```python
from build123d import *

# Parameters (mm, degrees)
SKETCH1_R           = 12
BOSS_EXTRUDE1_DEPTH = 31
FILLET1_R           = 1
SKETCH2_R           = 11.5
CUT_EXTRUDE1_DEPTH  = 1
SKETCH3_R           = 12.25
BOSS_EXTRUDE2_DEPTH = 20
FILLET2_R           = 0.5
SKETCH4_R           = 3.5
BOSS_EXTRUDE3_DEPTH = 3
SKETCH5_R           = 1.125510402
BOSS_EXTRUDE4_DEPTH = 9.5


with BuildPart() as part:
    # Sketch1 → Boss-Extrude1 (new body)
    with BuildSketch(Plane(origin=(0, 0, 0), x_dir=(0, 0, -1), z_dir=(1, 0, 0))):
        Circle(SKETCH1_R)
    extrude(amount=BOSS_EXTRUDE1_DEPTH)

    # Fillet1
    fillet1_edges = [part.edges().sort_by_distance(p)[0] for p in [
        (31, 0, 12),
    ]]
    fillet(fillet1_edges, radius=FILLET1_R)

    # Sketch2 → Cut-Extrude1 (cut)
    with BuildSketch(Plane.ZY):
        Circle(SKETCH2_R)
    extrude(amount=-CUT_EXTRUDE1_DEPTH, mode=Mode.SUBTRACT)

    # Sketch3 → Boss-Extrude2 (add)
    with BuildSketch(Plane(origin=(31, 0, 0), x_dir=(0, 0, -1), z_dir=(1, 0, 0))):
        Circle(SKETCH3_R)
    extrude(amount=BOSS_EXTRUDE2_DEPTH)

    # Fillet2
    fillet2_edges = [part.edges().sort_by_distance(p)[0] for p in [
        (31, 0, 12.25),
        (51, 0, 12.25),
    ]]
    fillet(fillet2_edges, radius=FILLET2_R)

    # Sketch4 → Boss-Extrude3 (add)
    with BuildSketch(Plane(origin=(51, 0, 0), x_dir=(0, 0, -1), z_dir=(1, 0, 0))):
        Circle(SKETCH4_R)
    extrude(amount=BOSS_EXTRUDE3_DEPTH)

    # Sketch5 → Boss-Extrude4 (add)
    with BuildSketch(Plane(origin=(54, 0, 0), x_dir=(0, 0, -1), z_dir=(1, 0, 0))):
        Circle(SKETCH5_R)
    extrude(amount=BOSS_EXTRUDE4_DEPTH)


solid = part.part
```
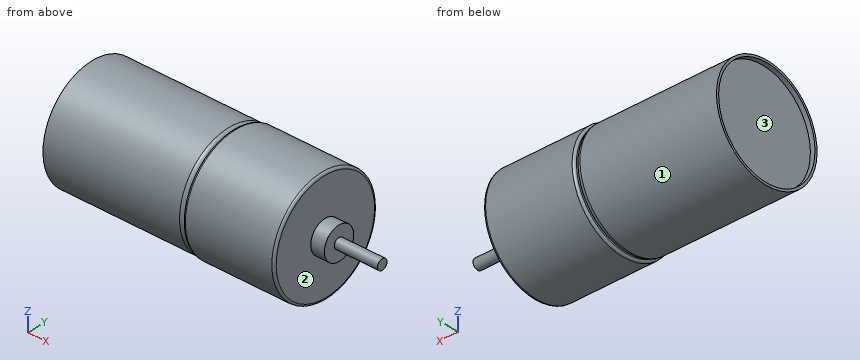
For this review, take the finished solid that the model builds, in its own axes (mm). Face numbers are marked on the shaded views. Give positions to 0.01 mm unless a question says otherwise; leave off trailing zeros. Loops run counter-clockwise (first coordinate to the right, second up) from the corner with the lowest first, then second, coordinate; pieces in that order, holes last. Notation, with made-up numbers: M -12.5,22 L 22.5,22 A34 ccw 22.5,58 Z; hole C 51,23.25 d1. An arc over 180 degrees is marked long. One line per item, written item: value. Start each with the question number.
Q1. Clearance check with flat-ended pins moving along their axes: pin 1 Ø10 at (y, z) = (9, 6) entering from +X; pin 2 Ø5 at (x, z) = (32.5, 3) entering from +Y; pin 3 Ø4 at (x, z) = (17, 0) entering from +Y. State where each tip first meets the part, or that it passes through.
Q2. For L1, parallel to Y at x = 0.3, z = 0; L2, parallel to X at y = 8, z = -5; L3, parallel to X at y = 0.5, z = 0.5, list the stretches that pass through material, from the lowest coordinate up.
Q3. Draft analysis for pull direction Y (two halves, no side actions). For the marked faces 1, 2 and 3, state which applies: released by +Y, released by -Y, zero draft, split by the parting line, or undercut.
Q4. Add section A-A (y = 0). Give the boundary of the cut face in (x, z), and give its area (3 significant figures).
Q5. Add section C-C (x = 8.5). Give the boundary of the cut face in (y, z).
Q6. Add section D-D (x = 56.5). Give the boundary of the cut face in (y, z), and give its area (3 significant figures).
Reply:
1. pin 1: x = 51
1. pin 2: y = 12.24
1. pin 3: y = 12
2. L1: -12 to -11.5, 11.5 to 12
2. L2: 1 to 51
2. L3: 1 to 63.5
3. face 1: split by the parting line
3. face 2: zero draft
3. face 3: undercut
4. outline: M 0,-12 L 30,-12 A1 ccw 31,-11 L 31,-11.75 A0.5 ccw 31.5,-12.25 L 50.5,-12.25 A0.5 ccw 51,-11.75 L 51,-3.5 L 54,-3.5 L 54,-1.13 L 63.5,-1.13 L 63.5,1.13 L 54,1.13 L 54,3.5 L 51,3.5 L 51,11.75 A0.5 ccw 50.5,12.25 L 31.5,12.25 A0.5 ccw 31,11.75 L 31,11 A1 ccw 30,12 L 0,12 L 0,11.5 L 1,11.5 L 1,-11.5 L 0,-11.5 Z
4. area: 1,250 mm²
5. outline: C 0,0 d24
6. outline: C 0,0 d2.25
6. area: 3.98 mm²
